Read the model definition and answer for the solid it produces. Units are mm, in the model's axes. A direction names the side the tool comes from. Give positions to 0.01 mm unless a question says otherwise; leave off trailing zeros. Loops run counter-clockwise (first coordinate to the right, second up) from the corner with the lowest first, then second, coordinate; pieces in that order, holes last. Notation, with made-up numbers: (46, 80) - (71, 80) arc R29 cw to (71, 101) - close; hole circle Ø5 at (14, 38). An arc over 180 degrees is marked (long way). Write item = value, one per line.
```python
from build123d import *

# Parameters (mm, degrees)
BOSS_EXTRUDE2_DEPTH = 91


with BuildPart() as part:
    # Sketch1 → Boss-Extrude2 (new body)
    with BuildSketch(Plane.XY):
        with BuildLine():
            ThreePointArc((364.5, 0), (-257.740421742, 257.740421742), (0, -364.5))
            ThreePointArc((0, -364.5), (257.740421742, -257.740421742), (364.5, 0))
        make_face()
        with BuildLine():
            Line((70, -150), (0, -150))
            Line((0, -150), (-70, -150))
            Line((-70, -150), (-70, -66.467106312))
            ThreePointArc((-70, -66.467106312), (-35.78292841, 89.651872573), (96.529147005, 0))
            ThreePointArc((96.529147005, 0), (89.651872573, -35.78292841), (70, -66.467106312))
            Line((70, -66.467106312), (70, -150))
        make_face(mode=Mode.SUBTRACT)
    extrude(amount=BOSS_EXTRUDE2_DEPTH)


solid = part.part
```
1) Each of these flat-tipped pins is pushed along its axis until it touches: P1, Ø10, axis at y = 95.5, z = 69.5, coming from the -X side; P2, Ø6, axis at x = -208.5, z = 46, coming from the +Y side; P3, Ø1, axis at x = 160.5, z = 45.5, coming from the -Y side. Where does it stop, or does it pass through?
Output:
P1 = -353.09
P2 = 301.05
P3 = -327.51
2) A tool of negligible diameter and unlimited length cuts with its end or side. For faces 4 (the face through (76, -76, 0)), 5 (the face through (1, -150, 45)), from which of +Z, -Z, +X, -X, +Y, -Y can it reach the whole face along a straight path? Write none if from no direction.
Output:
face_4 = -Z, +X, -X, +Y, -Y
face_5 = +Z, -Z
3) A cutting plane is placed at B-B on y = -35.5. Determine the outline of the cut face in (x, z), then the cut area to 3 significant figures.
Output:
outline = (-362.77, 0) - (-89.76, 0) - (-89.76, 91) - (-362.77, 91) - close; (89.76, 0) - (362.77, 0) - (362.77, 91) - (89.76, 91) - close
area = 49,700 mm²
4) The mould has two halves that part along Y. Classify faces 1 (the face through (70, -108, 45)), 2 (the face through (-70, -109, 45)), 3 (the face through (76, -76, 91)): pulls with the +Y half, pulls with the -Y half, needs draft (parallel to the pull), parting line crosses it, or undercut.
Output:
face_1 = undercut
face_2 = undercut
face_3 = needs draft
5) A cutting plane is placed at C-C on x = 35.5. Determine the outline of the cut face in (y, z).
Output:
outline = (-362.77, 0) - (-150, 0) - (-150, 91) - (-362.77, 91) - close; (89.76, 0) - (362.77, 0) - (362.77, 91) - (89.76, 91) - close
6) Find the intervals of material crossed by probe 1 along Y at (x, z) = (0, 30); probe 2 along Y at (x, z) = (87.5, 68.5); probe 3 along X at (y, z) = (-50, 32), in increasing order.
Output:
probe_1 = -364.5 to -150, 96.53 to 364.5
probe_2 = -353.84 to -40.76, 40.76 to 353.84
probe_3 = -361.05 to -82.57, 82.57 to 361.05
7) A cutting plane is placed at D-D on x = -222.5. Determine the outline of the cut face in (y, z), then the cut area to 3 significant figures.
Output:
outline = (-288.71, 0) - (288.71, 0) - (288.71, 91) - (-288.71, 91) - close
area = 52,500 mm²
8) A cutting plane is placed at A-A on z = 14.5. Determine the outline of the cut face in (x, y).
Output:
outline = circle Ø729 at (0, 0); hole (-70, -150) - (70, -150) - (70, -66.47) arc R96.53 ccw (long way) to (-70, -66.47) - close
